from build123d import *

# Parameters (mm, degrees)
SKETCH1_W           = 152.4
SKETCH1_H           = 152.4
BOSS_EXTRUDE1_DEPTH = 31.75
SKETCH2_R           = 6
CUT_EXTRUDE1_DEPTH  = 15
FILLET1_R           = 10
FILLET2_R           = 10


with BuildPart() as part:
    # Sketch1 → Boss-Extrude1 (new body)
    with BuildSketch(Plane(origin=(0, 0, 0), x_dir=(1, 0, 0), z_dir=(0, 1, 0))):
        with Locations((42.446979866, 76.2)):
            Rectangle(SKETCH1_W, SKETCH1_H)
    extrude(amount=BOSS_EXTRUDE1_DEPTH)

    # Sketch2 → Cut-Extrude1 (cut)
    with BuildSketch(Plane(origin=(0, 31.75, 0), x_dir=(1, 0, 0), z_dir=(0, 1, 0))):
        with Locations(Location((42.446979866, 76.2, 0), (0, 0, 270))):
            Circle(SKETCH2_R)
    extrude(amount=-CUT_EXTRUDE1_DEPTH, mode=Mode.SUBTRACT)

    # Fillet1
    fillet1_edges = [part.edges().sort_by_distance(p)[0] for p in [
        (118.646979866, 31.75, -76.2),
        (42.446979866, 31.75, -152.4),
        (-33.753020134, 31.75, -76.2),
        (42.446979866, 31.75, 0),
    ]]
    fillet(fillet1_edges, radius=FILLET1_R)

    # Fillet2
    fillet2_edges = [part.edges().sort_by_distance(p)[0] for p in [
        (42.446979866, 0, -152.4),
        (118.646979866, 0, -76.2),
        (42.446979866, 0, 0),
        (-33.753020134, 0, -76.2),
    ]]
    fillet(fillet2_edges, radius=FILLET2_R)


solid = part.part
Model file for the job. Use its own axes, mm. Give positions to 0.01 mm unless a question says otherwise; leave off trailing zeros. Loops run counter-clockwise (first coordinate to the right, second up) from the corner with the lowest first, then second, coordinate; pieces in that order, holes last. Notation, with made-up numbers: (66, -38.75) -> (72, -38.75) arc R9 ccw to (72, -27.75) -> close; hole circle Ø4 at (-2.5, 2). An arc over 180 degrees is marked (long way). Use a Markdown table: item, result. Add a question column.
(1) Slice it at D-D on z = -15. List the corners of the cut face in (x, y), and give its area (3 significant figures).
(2) Drop a flat-ended pin along its axis: pin 1 Ø1 at (x, y) = (51.5, 5.5) entering from -Z. Give the stop position or say it passes through.
(3) Mould opens along X. For faces 1 (the flat face through (43, 16.75, -76)), 2 (the flat face through (118.647, 16, -75)), 3 (the cylindrical face through (-30.901, 28.743, -77.267)), 4 (the cylindrical face through (36.59, 24.36, -77.5)) say: +X half, -X half, draft (parallel to the pull), parting line (faces both ways), or undercut.
(4) Slice it at C-C on y = 28. List the corners of the cut face in (x, z), and give its area (3 significant figures).
(5) Slice it at A-A on x = 6.5. List the corners of the cut face in (y, z).
(6) Slice it at B-B on z = -76.2. List the corners of the cut face in (x, y), and give its area (3 significant figures).
(7) Wall check: line 1 along X through (y, z) = (20.25, -76.2); line 2 along Z through (x, y) = (25.5, 22); line 3 along X through (y, z) = (27.5, -76.2). Give the ranges that are in metal, low to high.
Filled sheet:
| question | item | result |
|---|---|---|
| 1 | outline | (-33.75, 10) arc R10 ccw to (-23.75, 0) -> (108.65, 0) arc R10 ccw to (118.65, 10) -> (118.65, 21.75) arc R10 ccw to (108.65, 31.75) -> (-23.75, 31.75) arc R10 ccw to (-33.75, 21.75) -> close |
| 1 | area | 4,750 mm2 |
| 2 | pin 1 | z = -151.57 |
| 3 | face 1 | undercut |
| 3 | face 2 | +X half |
| 3 | face 3 | -X half |
| 3 | face 4 | undercut |
| 4 | outline | (-31.56, -150.21) -> (116.45, -150.21) -> (116.45, -2.19) -> (-31.56, -2.19) -> close; hole circle Ø12 at (42.45, -76.2) |
| 4 | area | 21,800 mm2 |
| 5 | outline | (0, -142.4) arc R10 ccw to (10, -152.4) -> (21.75, -152.4) arc R10 ccw to (31.75, -142.4) -> (31.75, -10) arc R10 ccw to (21.75, 0) -> (10, 0) arc R10 ccw to (0, -10) -> close |
| 6 | outline | (-33.75, 10) arc R10 ccw to (-23.75, 0) -> (108.65, 0) arc R10 ccw to (118.65, 10) -> (118.65, 21.75) arc R10 ccw to (108.65, 31.75) -> (48.45, 31.75) -> (48.45, 16.75) -> (36.45, 16.75) -> (36.45, 31.75) -> (-23.75, 31.75) arc R10 ccw to (-33.75, 21.75) -> close |
| 6 | area | 4,570 mm2 |
| 7 | line 1 | -33.75 to 36.45, 48.45 to 118.65 |
| 7 | line 2 | -152.4 to 0 |
| 7 | line 3 | -31.93 to 36.45, 48.45 to 116.83 |
